from build123d import *

# Parameters (mm, degrees)
CYLINDER045_R          = 1.7
CYLINDER045_DEPTH      = 20
CYLINDER045_ROLL_ANGLE = 90
CYLINDER044_R          = 1.7
CYLINDER044_DEPTH      = 20
CYLINDER044_ROLL_ANGLE = 90
CYLINDER043_R          = 1.7
CYLINDER043_DEPTH      = 20
CYLINDER043_ROLL_ANGLE = 90
CYLINDER040_R          = 1.7
CYLINDER040_DEPTH      = 20
CYLINDER040_ROLL_ANGLE = 90
CYLINDER041_R          = 1.7
CYLINDER041_DEPTH      = 20
CYLINDER041_ROLL_ANGLE = 90
CYLINDER042_R          = 1.7
CYLINDER042_DEPTH      = 20
CYLINDER042_ROLL_ANGLE = 90
SKETCH022_R            = 1.7
PAD020_DEPTH           = 20
SKETCH009_W            = 250
SKETCH009_H            = 420
SKETCH009_R            = 7.1
SKETCH009_R_2          = 1.3
SKETCH009_W_2          = 18
SKETCH009_H_2          = 7
PAD009_DEPTH           = 5


with BuildPart() as cylinder045:
    # Cylinder045 → Cylinder045 (new body)
    with BuildSketch(Plane.XY):
        Circle(CYLINDER045_R)
    extrude(amount=CYLINDER045_DEPTH)


with BuildPart() as cylinder045_1:
    # Cylinder045 roll: moved
    add(cylinder045.part.rotate(Axis((0, 0, 0), (1, 0, 0)), CYLINDER045_ROLL_ANGLE))


with BuildPart() as cylinder045_2:
    # Cylinder045 placement: moved
    add(cylinder045_1.part.moved(Location((-205, -140, 210))))


with BuildPart() as cylinder044:
    # Cylinder044 → Cylinder044 (new body)
    with BuildSketch(Plane.XY):
        Circle(CYLINDER044_R)
    extrude(amount=CYLINDER044_DEPTH)


with BuildPart() as cylinder044_1:
    # Cylinder044 roll: moved
    add(cylinder044.part.rotate(Axis((0, 0, 0), (1, 0, 0)), CYLINDER044_ROLL_ANGLE))


with BuildPart() as cylinder044_2:
    # Cylinder044 placement: moved
    add(cylinder044_1.part.moved(Location((-205, -140, 20))))


with BuildPart() as cylinder043:
    # Cylinder043 → Cylinder043 (new body)
    with BuildSketch(Plane.XY):
        Circle(CYLINDER043_R)
    extrude(amount=CYLINDER043_DEPTH)


with BuildPart() as cylinder043_1:
    # Cylinder043 roll: moved
    add(cylinder043.part.rotate(Axis((0, 0, 0), (1, 0, 0)), CYLINDER043_ROLL_ANGLE))


with BuildPart() as cylinder043_2:
    # Cylinder043 placement: moved
    add(cylinder043_1.part.moved(Location((-205, -140, 115))))


with BuildPart() as cylinder040:
    # Cylinder040 → Cylinder040 (new body)
    with BuildSketch(Plane.XY):
        Circle(CYLINDER040_R)
    extrude(amount=CYLINDER040_DEPTH)


with BuildPart() as cylinder040_1:
    # Cylinder040 roll: moved
    add(cylinder040.part.rotate(Axis((0, 0, 0), (1, 0, 0)), CYLINDER040_ROLL_ANGLE))


with BuildPart() as cylinder040_2:
    # Cylinder040 placement: moved
    add(cylinder040_1.part.moved(Location((205, -135, 20))))


with BuildPart() as cylinder041:
    # Cylinder041 → Cylinder041 (new body)
    with BuildSketch(Plane.XY):
        Circle(CYLINDER041_R)
    extrude(amount=CYLINDER041_DEPTH)


with BuildPart() as cylinder041_1:
    # Cylinder041 roll: moved
    add(cylinder041.part.rotate(Axis((0, 0, 0), (1, 0, 0)), CYLINDER041_ROLL_ANGLE))


with BuildPart() as cylinder041_2:
    # Cylinder041 placement: moved
    add(cylinder041_1.part.moved(Location((205, -135, 115))))


with BuildPart() as cylinder042:
    # Cylinder042 → Cylinder042 (new body)
    with BuildSketch(Plane.XY):
        Circle(CYLINDER042_R)
    extrude(amount=CYLINDER042_DEPTH)


with BuildPart() as cylinder042_1:
    # Cylinder042 roll: moved
    add(cylinder042.part.rotate(Axis((0, 0, 0), (1, 0, 0)), CYLINDER042_ROLL_ANGLE))


with BuildPart() as cylinder042_2:
    # Cylinder042 placement: moved
    add(cylinder042_1.part.moved(Location((205, -135, 210))))


with BuildPart() as fusion014:
    # Sketch022 → Pad020 (new body)
    with BuildSketch(Plane.XZ.offset(135)):
        with Locations((-150, -5)):
            Circle(SKETCH022_R)
        with Locations((0, -5)):
            Circle(SKETCH022_R)
        with Locations((150, -5)):
            Circle(SKETCH022_R)
    extrude(amount=PAD020_DEPTH)

    # Fusion014: union Cylinder045, Cylinder044, Cylinder043, Cylinder040, Cylinder041, Cylinder042
    add(cylinder045_2.part)
    add(cylinder044_2.part)
    add(cylinder043_2.part)
    add(cylinder040_2.part)
    add(cylinder041_2.part)
    add(cylinder042_2.part)


with BuildPart() as cut017:
    # Sketch009 → Pad009 (new body)
    with BuildSketch(Plane(origin=(-160, -140, 200), x_dir=(0, 0, -1), z_dir=(0, -1, 0))):
        with Locations((85, 160.000183)):
            Rectangle(SKETCH009_W, SKETCH009_H)
        with Locations((11.81, 19.93)):
            Circle(SKETCH009_R, mode=Mode.SUBTRACT)
        with Locations((11.81, 39.93)):
            Circle(SKETCH009_R, mode=Mode.SUBTRACT)
        with Locations((11.81, 59.93)):
            Circle(SKETCH009_R, mode=Mode.SUBTRACT)
        with Locations((11.81, 79.93)):
            Circle(SKETCH009_R, mode=Mode.SUBTRACT)
        with Locations((11.81, 99.93)):
            Circle(SKETCH009_R, mode=Mode.SUBTRACT)
        with Locations((11.81, 119.93)):
            Circle(SKETCH009_R, mode=Mode.SUBTRACT)
        with Locations((11.81, 146.89)):
            Circle(SKETCH009_R, mode=Mode.SUBTRACT)
        with Locations((11.81, 166.89)):
            Circle(SKETCH009_R, mode=Mode.SUBTRACT)
        with Locations((11.81, 186.89)):
            Circle(SKETCH009_R, mode=Mode.SUBTRACT)
        with Locations((11.81, 246.89)):
            Circle(SKETCH009_R, mode=Mode.SUBTRACT)
        with Locations((109.58, 246.89)):
            Circle(SKETCH009_R, mode=Mode.SUBTRACT)
        with Locations((11.81, 226.89)):
            Circle(SKETCH009_R, mode=Mode.SUBTRACT)
        with Locations((11.81, 206.89)):
            Circle(SKETCH009_R, mode=Mode.SUBTRACT)
        with Locations((109.58, 186.89)):
            Circle(SKETCH009_R, mode=Mode.SUBTRACT)
        with Locations((109.58, 226.89)):
            Circle(SKETCH009_R, mode=Mode.SUBTRACT)
        with Locations((109.58, 206.89)):
            Circle(SKETCH009_R, mode=Mode.SUBTRACT)
        with Locations((109.58, 166.89)):
            Circle(SKETCH009_R, mode=Mode.SUBTRACT)
        with Locations((109.63, 146.89)):
            Circle(SKETCH009_R, mode=Mode.SUBTRACT)
        with Locations((109.63, 119.95)):
            Circle(SKETCH009_R, mode=Mode.SUBTRACT)
        with Locations((109.63, 99.95)):
            Circle(SKETCH009_R, mode=Mode.SUBTRACT)
        with Locations((109.63, 79.95)):
            Circle(SKETCH009_R, mode=Mode.SUBTRACT)
        with Locations((109.63, 59.95)):
            Circle(SKETCH009_R, mode=Mode.SUBTRACT)
        with Locations((109.63, 39.95)):
            Circle(SKETCH009_R, mode=Mode.SUBTRACT)
        with Locations((109.63, 19.95)):
            Circle(SKETCH009_R, mode=Mode.SUBTRACT)
        with Locations((5.9944, 5.9944)):
            Circle(SKETCH009_R_2, mode=Mode.SUBTRACT)
        with Locations((5.9944, 134)):
            Circle(SKETCH009_R_2, mode=Mode.SUBTRACT)
        with Locations((5.9944, 269.79)):
            Circle(SKETCH009_R_2, mode=Mode.SUBTRACT)
        with Locations((115, 269.79)):
            Circle(SKETCH009_R_2, mode=Mode.SUBTRACT)
        with Locations((115, 5.9944)):
            Circle(SKETCH009_R_2, mode=Mode.SUBTRACT)
        with Locations((115, 134)):
            Circle(SKETCH009_R_2, mode=Mode.SUBTRACT)
        with Locations((42.87, 23.07)):
            Rectangle(SKETCH009_W_2, SKETCH009_H_2, mode=Mode.SUBTRACT)
        with Locations((42.87, 62.97)):
            Rectangle(SKETCH009_W_2, SKETCH009_H_2, mode=Mode.SUBTRACT)
        with Locations((42.87, 82.88)):
            Rectangle(SKETCH009_W_2, SKETCH009_H_2, mode=Mode.SUBTRACT)
        with Locations((42.87, 42.9)):
            Rectangle(SKETCH009_W_2, SKETCH009_H_2, mode=Mode.SUBTRACT)
        with Locations((42.87, 149.86)):
            Rectangle(SKETCH009_W_2, SKETCH009_H_2, mode=Mode.SUBTRACT)
        with Locations((42.87, 122.96)):
            Rectangle(SKETCH009_W_2, SKETCH009_H_2, mode=Mode.SUBTRACT)
        with Locations((42.87, 102.93)):
            Rectangle(SKETCH009_W_2, SKETCH009_H_2, mode=Mode.SUBTRACT)
        with Locations((42.87, 169.86)):
            Rectangle(SKETCH009_W_2, SKETCH009_H_2, mode=Mode.SUBTRACT)
        with Locations((42.87, 209.84)):
            Rectangle(SKETCH009_W_2, SKETCH009_H_2, mode=Mode.SUBTRACT)
        with Locations((42.87, 189.89)):
            Rectangle(SKETCH009_W_2, SKETCH009_H_2, mode=Mode.SUBTRACT)
        with Locations((42.87, 250.02)):
            Rectangle(SKETCH009_W_2, SKETCH009_H_2, mode=Mode.SUBTRACT)
        with Locations((42.870057, 229.9)):
            Rectangle(SKETCH009_W_2, SKETCH009_H_2, mode=Mode.SUBTRACT)
        with Locations((77.82, 22.87)):
            Rectangle(SKETCH009_W_2, SKETCH009_H_2, mode=Mode.SUBTRACT)
        with Locations((77.335221, 42.83)):
            Rectangle(SKETCH009_W_2, SKETCH009_H_2, mode=Mode.SUBTRACT)
        with Locations((77.692519, 62.9)):
            Rectangle(SKETCH009_W_2, SKETCH009_H_2, mode=Mode.SUBTRACT)
        with Locations((77.789409, 82.84)):
            Rectangle(SKETCH009_W_2, SKETCH009_H_2, mode=Mode.SUBTRACT)
        with Locations((77.732999, 102.77)):
            Rectangle(SKETCH009_W_2, SKETCH009_H_2, mode=Mode.SUBTRACT)
        with Locations((77.819954, 122.86)):
            Rectangle(SKETCH009_W_2, SKETCH009_H_2, mode=Mode.SUBTRACT)
        with Locations((77.899539, 149.871817)):
            Rectangle(SKETCH009_W_2, SKETCH009_H_2, mode=Mode.SUBTRACT)
        with Locations((77.773082, 169.767253)):
            Rectangle(SKETCH009_W_2, SKETCH009_H_2, mode=Mode.SUBTRACT)
        with Locations((77.780992, 189.89)):
            Rectangle(SKETCH009_W_2, SKETCH009_H_2, mode=Mode.SUBTRACT)
        with Locations((77.671681, 209.83816)):
            Rectangle(SKETCH009_W_2, SKETCH009_H_2, mode=Mode.SUBTRACT)
        with Locations((77.692731, 229.7)):
            Rectangle(SKETCH009_W_2, SKETCH009_H_2, mode=Mode.SUBTRACT)
        with Locations((77.82, 250.02)):
            Rectangle(SKETCH009_W_2, SKETCH009_H_2, mode=Mode.SUBTRACT)
        with BuildLine():
            ThreePointArc((181.567028, 204.22761), (166.567028, 219.22761), (151.567028, 204.22761))
            Line((151.567028, 204.22761), (151.567028, 104.22761))
            ThreePointArc((151.567028, 104.22761), (166.567028, 89.22761), (181.567028, 104.22761))
            Line((181.567028, 204.22761), (181.567028, 104.22761))
        make_face(mode=Mode.SUBTRACT)
    extrude(amount=PAD009_DEPTH)

    # Cut017: cut Fusion014
    add(fusion014.part, mode=Mode.SUBTRACT)


solid = cut017.part
Source: CAD feature listing. Evaluate the final solid. Frame: model axes, mm. A direction names the side the tool comes from. Round coordinates to 2 decimals unless told otherwise and drop trailing zeros. Loops run counter-clockwise (first coordinate to the right, second up) from the corner with the lowest first, then second, coordinate; pieces in that order, holes last. Notation, with made-up numbers: (83.5, 17.5) -> (122.5, 17.5) arc R26 ccw to (122.5, 38.5) -> close; hole circle Ø1 at (69, -29.75). An arc over 180 degrees is marked (long way). Answer as a JSON object with one key per item and string values. Group by question number.
Q1. Mould query, pull axis Z, two halves, no side actions, for faces 3 (the cylindrical face through (-99.758, -142.465, 195.283)), 4 (the flat face through (3, -140, 117)). Classes: pulls with the +Z half, pulls with the -Z half, needs draft (parallel to the pull), parting line crosses it, or undercut.
Q2. Section query B-B (z = 37.5). Output: boundary loops of the cut face in (x, y).
Q3. Access query for faces 1 (the flat face through (3, -145, 117)), 2 (the cylindrical face through (-70.77, -142.46, 33.76)). Directions: +Z, -Z, +X, -X, +Y, -Y. A direction counts if a zero-diameter tool reaches every point of the face in a straight line with its end or side. Return the directions, or none.
Q4. Ray query, line 1 (X direction, y = -140.8, z = 35); line 2 (Z direction, x = -37, y = -143.1); line 3 (Z direction, x = -5, y = -142.35). Return the intervals inside material, ascending. Write a range as from..to.
Q5. Contact query for a flat-ended pin moving along its axis: P1, Ø2, axis at x = 0, z = -5, coming from the -Y side. Output: stop coordinate, or through.
Q6. Section query A-A (z = 188.19). State how many separate pieces and enclosed holes the cut face has, plus the area to 3 significant figures.
Completed:
{
 "1": {"face 3": "undercut", "face 4": "needs draft"},
 "2": {"outline": "(-210, -145) -> (-70.21, -145) -> (-70.21, -140) -> (-210, -140) -> close; (58.67, -145) -> (210, -145) -> (210, -140) -> (58.67, -140) -> close"},
 "3": {"face 1": "+Z, -Z, +X, -X, -Y", "face 2": "+Y, -Y"},
 "4": {"line 1": "-210..-70.69, 59.15..210", "line 2": "-10..18.43, 48.43..83.96, 96.78..113.18, 131.18..148.13, 166.13..181.79, 194.59..240", "line 3": "-10..18.43, 48.43..240"},
 "5": {"P1": "through"},
 "6": {"separate pieces": "13", "enclosed holes": "0", "area": "1,250 mm²"}
}
